Design review of the part built by this model. Coordinates are the model's own, in mm. A direction names the side the tool comes from. Give positions to 0.01 mm unless a question says otherwise; leave off trailing zeros. Loops run counter-clockwise (first coordinate to the right, second up) from the corner with the lowest first, then second, coordinate; pieces in that order, holes last. Notation, with made-up numbers: M -21.5,58 L 30.5,58 A21 ccw 30.5,65 Z; hole C 8.25,46 d10. An arc over 180 degrees is marked long. Answer as CSV lines item,"result".
```python
from build123d import *

# Parameters (mm, degrees)
F2_SIZE2 = 5.08
F2_SIZE  = 5.08
F3_R     = 5.08
F4_SIZE  = 5.08


with BuildPart() as f1:
    # F0 (on Top) → F1 (revolve)
    with BuildSketch(Plane.XY):
        Polygon((0, 25.4), (0, 0), (76.2, 0), (76.2, 20.32), (30.48, 20.32), (30.48, 40.64), (12.7, 40.64), (12.7, 25.4), align=None)
    revolve(axis=Axis((38.1, 0, 0), (-1, 0, 0)))

    # F2
    f2_edges = [f1.edges().sort_by_distance(p)[0] for p in [
        (76.2, -20.32, 0),
    ]]
    chamfer(f2_edges, length=F2_SIZE, length2=F2_SIZE2)

    # F3
    f3_edges = [f1.edges().sort_by_distance(p)[0] for p in [
        (12.7, -40.64, 0),
        (30.48, -40.64, 0),
    ]]
    fillet(f3_edges, radius=F3_R)

    # F4
    f4_edges = [f1.edges().sort_by_distance(p)[0] for p in [
        (0, -25.4, 0),
    ]]
    chamfer(f4_edges, length=F4_SIZE)


solid = f1.part
```
1. We need section D-D, the plane x = 29. Write out the cut boundary in (y, z), plus the area to 3 significant figures.
Answer block:
outline,"C 0,0 d78.29"
area,"4,810 mm²"
2. To check wall thickness, follow L1, parallel to X at y = 13, z = 30; L2, parallel to Y at x = 27, z = -21; L3, parallel to Y at x = 21, z = -18.5. State the ranges of each line that lie inside material, in increasing order. Write a range as [from, to].
Answer block:
L1,"[12.7, 30.48]"
L2,"[-34.49, 34.49]"
L3,"[-36.19, 36.19]"
3. For P1, Ø6, axis at x = 55, y = 11, coming from the -Z side; P2, Ø12, axis at y = -29, z = 15.5, coming from the +X side; P3, Ø4, axis at x = 25.5, z = 5.5, coming from the +Y side, all flat-tipped, find the tip position at first contact; note any pin that passes through.
Answer block:
P1,"z = -18.68"
P2,"x = 30.48"
P3,"y = 40.49"
4. We need section A-A, the plane y = 0. Write out the cut boundary in (x, z).
Answer block:
outline,"M 0,-20.32 L 5.08,-25.4 L 12.7,-25.4 L 12.7,-35.56 A5.08 ccw 17.78,-40.64 L 25.4,-40.64 A5.08 ccw 30.48,-35.56 L 30.48,-20.32 L 71.12,-20.32 L 76.2,-15.24 L 76.2,15.24 L 71.12,20.32 L 30.48,20.32 L 30.48,35.56 A5.08 ccw 25.4,40.64 L 17.78,40.64 A5.08 ccw 12.7,35.56 L 12.7,25.4 L 5.08,25.4 L 0,20.32 Z"
5. We need section C-C, the plane x = 61. Write out the cut boundary in (y, z).
Answer block:
outline,"C 0,0 d40.64"
6. For faces 1 (the cylindrical face through (8.837, -5.506, 24.796)), 2 (the cylindrical face through (21.537, -5.291, -40.294)), 3 (the cylindrical face through (50.516, -2.645, -20.147)), list the 3-axis set-ups (+Z, -Z, +X, -X, +Y, -Y) from which the entire face can be reached by the end or side of a thin tool; tool diameter is ignored.
Answer block:
face 1,"-X"
face 2,"+X, -X"
face 3,"+X"
